Geometry check sheet. Reference: the model listing, model coordinates, mm. Give positions to 0.01 mm unless a question says otherwise; leave off trailing zeros. Order: outer loops, then holes, each group sorted by start corner. A loop starts at its lowest first (then second) coordinate and runs counter-clockwise, first axis right, second up. Notation, with made-up numbers: M -11.75,-22 L 23.25,-22 A27 ccw 23.25,-6 Z; hole C -16,50 d4. An arc over 180 degrees is marked long. Answer as CSV lines item,"result". Start each with the question number.
Q1. Section check A-A, the plane y = 18.5. Record the boundary of the cut face in (x, z).
Q2. Section check B-B, the plane z = -0.5. Record the boundary of the cut face in (x, y).
Q3. Section check D-D, the plane z = 1.5. Record the boundary of the cut face in (x, y).
Q4. Section check C-C, the plane x = -2.75. Record the boundary of the cut face in (y, z).
Q5. Go/stop test with flat-tipped pins: pin 1 (1 mm diameter, centred on y = 12, z = -0.5, fed in from +X); pin 2 (0.6 mm diameter, centred on y = 18, z = -1.5, fed in from -X); pin 3 (1.5 mm diameter, centred on x = 0, y = 19.5, fed in from +Z); pin 4 (2 mm diameter, centred on x = -2, z = 1.5, fed in from +Y). Record where each tip stops, or that it passes through.
Q6. Thickness scan on line 1 (Z direction, x = 2, y = 18); line 2 (Y direction, x = -3, z = -0.5); line 3 (Z direction, x = -0.5, y = 20.5). Record the ranges inside material, lowest first.
```python
from build123d import *

# Parameters (mm, degrees)
F1_DEPTH = 20
F2_W     = 1.9
F2_H     = 1.3
F2_W_2   = 1.3
F2_H_2   = 1.9
F3_DEPTH = 30


with BuildPart() as f1:
    # F0 (on Front) → F1 (new body)
    with BuildSketch(Plane.XZ):
        Polygon((3.75, 0.0170362348), (1.8602461879, 3.2561133816), (-1.8897538121, 3.2390771468), (-3.75, -0.0170362348), (-1.8602461879, -3.2561133816), (1.8897538121, -3.2390771468), align=None)
    extrude(amount=F1_DEPTH)

    # F2 (on Front) → F3 (join)
    with BuildSketch(Plane.XZ):
        with Locations((0, 1.6)):
            Rectangle(F2_W, F2_H)
        with Locations((-1.6, 0)):
            Rectangle(F2_W_2, F2_H_2)
        Rectangle(F2_W, F2_H_2)
        with Locations((1.6, 0)):
            Rectangle(F2_W_2, F2_H_2)
        with Locations((0, -1.6)):
            Rectangle(F2_W, F2_H)
    extrude(amount=-F3_DEPTH)


solid = f1.part
```
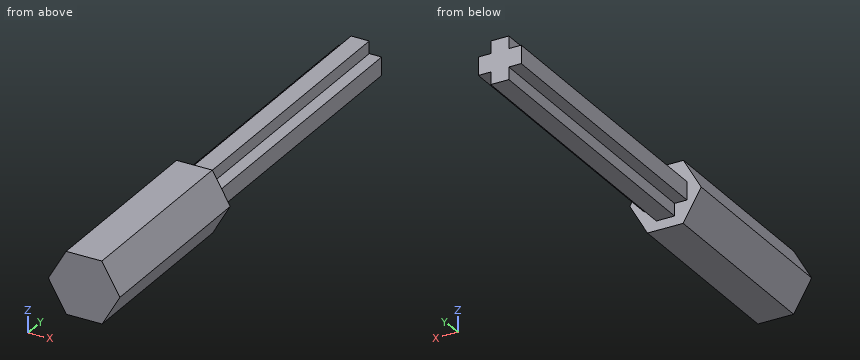
Answer block:
1,outline,"M -2.25,-0.95 L -0.95,-0.95 L -0.95,-2.25 L 0.95,-2.25 L 0.95,-0.95 L 2.25,-0.95 L 2.25,0.95 L 0.95,0.95 L 0.95,2.25 L -0.95,2.25 L -0.95,0.95 L -2.25,0.95 Z"
2,outline,"M -3.47,-20 L 3.45,-20 L 3.45,0 L 2.25,0 L 2.25,30 L -2.25,30 L -2.25,0 L -3.47,0 Z"
3,outline,"M -2.88,-20 L 2.88,-20 L 2.88,0 L 0.95,0 L 0.95,30 L -0.95,30 L -0.95,0 L -2.88,0 Z"
4,outline,"M -20,-1.73 L 0,-1.73 L 0,1.73 L -20,1.73 Z"
5,pin 1,"stops at x = 2.25"
5,pin 2,"stops at x = -0.95"
5,pin 3,"stops at z = 2.25"
5,pin 4,"stops at y = 30"
6,line 1,"z = -0.95 to 0.95"
6,line 2,"y = -20 to 0"
6,line 3,"z = -2.25 to 2.25"
